The listing builds one solid part. Answer for the finished solid, in the listing's coordinates (mm). A direction names the side the tool comes from. Coordinates: 2 decimals unless noted, no trailing zeros. Order: outer loops, then holes, each group sorted by start corner. A loop starts at its lowest first (then second) coordinate and runs counter-clockwise, first axis right, second up. Notation, with made-up numbers: (2.5, 72) - (18.5, 72) arc R26 ccw to (18.5, 108) - close; hole circle Ø7 at (32.5, 10). An arc over 180 degrees is marked (long way). Use a Markdown table: item, result. Add a question column.
Item 1: Flat-ended cylindrical pins translate along their axes: P1, Ø2, axis at y = 1, z = 4, coming from the +X side; P2, Ø2, axis at x = -4.5, z = 0.5, coming from the +Y side; P3, Ø1.5, axis at x = -5, z = 2.5, coming from the +Y side. Find the tip coordinate at first contact, or state that the pin passes through.
Item 2: Find the intervals of material crossed by line 1 along Z through (x, y) = (-3, 5.5); line 2 along Y through (x, z) = (-0.5, 3.6); line 3 along X through (y, z) = (-1, 3.45), in increasing order.
Item 3: The part is cut by section A-A, the plane z = 4.45. Give the vertices of the cut face in (x, y).
Item 4: For faces 5 (the flat face through (3, 0, 2.2)), 6 (the flat face through (2, -3, 2.6)), 7 (the flat face through (-3, -2, 2.6)), 8 (the flat face through (5, -5, 2)), 9 (the flat face through (0, 0, 0)), determine the directions among +Z, -Z, +X, -X, +Y, -Y from which every point of the face is accessible in a straight line to the end or side of a thin tool.
Item 5: The mould has two halves that part along Y. Classify faces 1 (the flat face through (3, 2, 2.6)), 2 (the cylindrical face through (1.6, -3, 4)), 3 (the cylindrical face through (-2.38, -10.74, 1.49)), 4 (the cylindrical face through (-3, -1.6, 4)): released by +Y, released by -Y, zero draft, split by the parting line, or undercut.
from build123d import *
from build123d import SkipClean  # not in build123d's __all__

# Parameters (mm, degrees)
F0_R     = 11
F1_DEPTH = 2
F2_SIZE  = 1
F3_R     = 6
F4_DEPTH = 0.2
F6_DEPTH = 3.2
F7_DEPTH = 0.4


with BuildPart() as f1:
    # F0 (on Top) → F1 (new body)
    with BuildSketch(Plane.XY):
        Circle(F0_R)
    extrude(amount=F1_DEPTH)

    # F2
    f2_edges = [f1.edges().sort_by_distance(p)[0] for p in [
        (-11, 0, 0),
    ]]
    chamfer(f2_edges, length=F2_SIZE)

    # F3 (on face) → F4 (join)
    with BuildSketch(Plane.XY.offset(2)):
        Circle(F3_R)
    extrude(amount=F4_DEPTH)

    # F5 (on face) → F6 (join)
    with BuildSketch(Plane.XY.offset(2.2)):
        with BuildLine():
            ThreePointArc((-0.0052788349, 3.7000174165), (0.3973518743, 4.0973692908), (0, 4.5))
            ThreePointArc((0, 4.5), (-0.0556126102, 4.4996563466), (-0.1112167263, 4.4986254389))
            ThreePointArc((-0.1112167263, 4.4986254389), (-2.6104676107, 2.9421967987), (-2.5, 0))
            ThreePointArc((-2.5, 0), (-2.4073466074, 0.6743013511), (-2.1362541503, 1.2986216559))
            ThreePointArc((-2.1362541503, 1.2986216559), (-1.6153328632, 2.9825624536), (-0.0052788349, 3.7000174165))
        make_face()
        with BuildLine():
            ThreePointArc((3.7000174165, 0.0052788349), (4.0973692908, -0.3973518743), (4.5, 0))
            ThreePointArc((4.5, 0), (4.4996563466, 0.0556126102), (4.4986254389, 0.1112167263))
            ThreePointArc((4.4986254389, 0.1112167263), (2.9421967987, 2.6104676107), (0, 2.5))
            ThreePointArc((0, 2.5), (0.6743013511, 2.4073466074), (1.2986216559, 2.1362541503))
            ThreePointArc((1.2986216559, 2.1362541503), (2.9825624536, 1.6153328632), (3.7000174165, 0.0052788349))
        make_face()
        with BuildLine():
            ThreePointArc((0, -4.5), (0.0556126102, -4.4996563466), (0.1112167263, -4.4986254389))
            ThreePointArc((0.1112167263, -4.4986254389), (2.6104676107, -2.9421967987), (2.5, 0))
            ThreePointArc((2.5, 0), (2.4073466074, -0.6743013511), (2.1362541503, -1.2986216559))
            ThreePointArc((2.1362541503, -1.2986216559), (1.6153328632, -2.9825624536), (0.0052788349, -3.7000174165))
            ThreePointArc((0.0052788349, -3.7000174165), (-0.3973518743, -4.0973692908), (0, -4.5))
        make_face()
        with BuildLine():
            ThreePointArc((-4.5, 0), (-4.4996563466, -0.0556126102), (-4.4986254389, -0.1112167263))
            ThreePointArc((-4.4986254389, -0.1112167263), (-2.9421967987, -2.6104676107), (0, -2.5))
            ThreePointArc((0, -2.5), (-0.6743013511, -2.4073466074), (-1.2986216559, -2.1362541503))
            ThreePointArc((-1.2986216559, -2.1362541503), (-2.9825624536, -1.6153328632), (-3.7000174165, -0.0052788349))
            ThreePointArc((-3.7000174165, -0.0052788349), (-4.0973692908, 0.3973518743), (-4.5, 0))
        make_face()
        with BuildLine():
            ThreePointArc((1.2986216559, 2.1362541503), (0.6743013511, 2.4073466074), (0, 2.5))
            ThreePointArc((0, 2.5), (-1.2254480528, 2.1790541686), (-2.1362541503, 1.2986216559))
            ThreePointArc((-2.1362541503, 1.2986216559), (-2.4073466074, 0.6743013511), (-2.5, 0))
            ThreePointArc((-2.5, 0), (-2.1790541686, -1.2254480528), (-1.2986216559, -2.1362541503))
            ThreePointArc((-1.2986216559, -2.1362541503), (-0.6743013511, -2.4073466074), (0, -2.5))
            ThreePointArc((0, -2.5), (1.2254480528, -2.1790541686), (2.1362541503, -1.2986216559))
            ThreePointArc((2.1362541503, -1.2986216559), (2.4073466074, -0.6743013511), (2.5, 0))
            ThreePointArc((2.5, 0), (2.1790541686, 1.2254480528), (1.2986216559, 2.1362541503))
        make_face()
    extrude(amount=F6_DEPTH)

    # F5 (on face) → F7 (cut)
    with BuildSketch(Plane.XY.offset(2.2)):
        with BuildLine():
            ThreePointArc((-4.5, 0), (-4.4996563466, -0.0556126102), (-4.4986254389, -0.1112167263))
            ThreePointArc((-4.4986254389, -0.1112167263), (-2.9421967987, -2.6104676107), (0, -2.5))
            ThreePointArc((0, -2.5), (-0.6743013511, -2.4073466074), (-1.2986216559, -2.1362541503))
            ThreePointArc((-1.2986216559, -2.1362541503), (-2.9825624536, -1.6153328632), (-3.7000174165, -0.0052788349))
            ThreePointArc((-3.7000174165, -0.0052788349), (-4.0973692908, 0.3973518743), (-4.5, 0))
        make_face()
        with BuildLine():
            ThreePointArc((-0.0052788349, 3.7000174165), (0.3973518743, 4.0973692908), (0, 4.5))
            ThreePointArc((0, 4.5), (-0.0556126102, 4.4996563466), (-0.1112167263, 4.4986254389))
            ThreePointArc((-0.1112167263, 4.4986254389), (-2.6104676107, 2.9421967987), (-2.5, 0))
            ThreePointArc((-2.5, 0), (-2.4073466074, 0.6743013511), (-2.1362541503, 1.2986216559))
            ThreePointArc((-2.1362541503, 1.2986216559), (-1.6153328632, 2.9825624536), (-0.0052788349, 3.7000174165))
        make_face()
        with BuildLine():
            ThreePointArc((3.7000174165, 0.0052788349), (4.0973692908, -0.3973518743), (4.5, 0))
            ThreePointArc((4.5, 0), (4.4996563466, 0.0556126102), (4.4986254389, 0.1112167263))
            ThreePointArc((4.4986254389, 0.1112167263), (2.9421967987, 2.6104676107), (0, 2.5))
            ThreePointArc((0, 2.5), (0.6743013511, 2.4073466074), (1.2986216559, 2.1362541503))
            ThreePointArc((1.2986216559, 2.1362541503), (2.9825624536, 1.6153328632), (3.7000174165, 0.0052788349))
        make_face()
        with BuildLine():
            ThreePointArc((0, -4.5), (0.0556126102, -4.4996563466), (0.1112167263, -4.4986254389))
            ThreePointArc((0.1112167263, -4.4986254389), (2.6104676107, -2.9421967987), (2.5, 0))
            ThreePointArc((2.5, 0), (2.4073466074, -0.6743013511), (2.1362541503, -1.2986216559))
            ThreePointArc((2.1362541503, -1.2986216559), (1.6153328632, -2.9825624536), (0.0052788349, -3.7000174165))
            ThreePointArc((0.0052788349, -3.7000174165), (-0.3973518743, -4.0973692908), (0, -4.5))
        make_face()
    with SkipClean():  # cleaning this boolean's faces spoils the solid; the shape is the same uncleaned
        extrude(amount=F7_DEPTH, mode=Mode.SUBTRACT)


solid = f1.part
Solution:
| question | item | result |
|---|---|---|
| 1 | P1 | stops at x = 4.5 |
| 1 | P2 | stops at y = 10.38 |
| 1 | P3 | stops at y = 10.06 |
| 2 | line 1 | z = 0 to 2 |
| 2 | line 2 | y = -2.75 to 2.45, 3.65 to 4.46 |
| 2 | line 3 | x = -4.33 to -3.46, -2.29 to 2.9 |
| 3 | outline | (-4.5, -0.11) arc R2.93 ccw to (0, -2.5) arc R2.5 ccw to (2.14, -1.3) arc R2.13 cw to (0.01, -3.7) arc R0.4 ccw to (0, -4.5) arc R4.5 ccw to (0.11, -4.5) arc R2.93 ccw to (2.5, 0) arc R2.5 ccw to (1.3, 2.14) arc R2.13 cw to (3.7, 0.01) arc R0.4 ccw to (4.5, 0) arc R4.5 ccw to (4.5, 0.11) arc R2.93 ccw to (0, 2.5) arc R2.5 ccw to (-2.14, 1.3) arc R2.13 cw to (-0.01, 3.7) arc R0.4 ccw to (0, 4.5) arc R4.5 ccw to (-0.11, 4.5) arc R2.93 ccw to (-2.5, 0) arc R2.5 ccw to (-1.3, -2.14) arc R2.13 cw to (-3.7, -0.01) arc R0.4 ccw to (-4.5, 0) arc R4.5 ccw to start |
| 4 | face 5 | none |
| 4 | face 6 | +X, -Y |
| 4 | face 7 | -X, -Y |
| 4 | face 8 | +Z |
| 4 | face 9 | -Z, +X, -X, +Y, -Y |
| 5 | face 1 | zero draft |
| 5 | face 2 | undercut |
| 5 | face 3 | split by the parting line |
| 5 | face 4 | undercut |
